```python
from build123d import *

# Parameters (mm, degrees)
SKETCH_1_W          = 0.3
SKETCH_1_H          = 1.5
SKETCH_1_R          = 2.5
SKETCH_1_R_2        = 1.5
EXTRUDE_1_DEPTH     = 15.2
SKETCH_1_4_W        = 0.3
SKETCH_1_4_H        = 1.5
EXTRUDE_2_DEPTH     = 2
CUT_EXTRUDE_2_DEPTH = 19.763794925
FILLET_1_R          = 0.4
SKETCH_1_5_R        = 2.5
SKETCH_1_5_R_2      = 1.5
EXTRUDE_3_DEPTH     = 1.2
CUT_EXTRUDE_START   = -1.2
SKETCH_1_7_R        = 1.5
CUT_EXTRUDE_1_DEPTH = 0.6
FILLET_2_R          = 0.4
SKETCH_3_R          = 2
EXTRUDE_4_DEPTH     = 0.5
SKETCH_3_3_R        = 0.5
EXTRUDE_5_DEPTH     = 6.5


with BuildPart() as part:
    # 草图1 → 凸台-拉伸1 (new body)
    # profile 1 of 5: a face of its own
    with BuildSketch(Plane.XY):
        with BuildLine():
            ThreePointArc((-6, 0), (-5.286764074, -2.837274331), (-3.31662479, -5))
            Line((-3.31662479, -5), (3.31662479, -5))
            ThreePointArc((3.31662479, -5), (5.286764074, -2.837274331), (6, 0))
            ThreePointArc((6, 0), (5.286764074, 2.837274331), (3.31662479, 5))
            Line((3.31662479, 5), (-3.31662479, 5))
            ThreePointArc((-3.31662479, 5), (-5.286764074, 2.837274331), (-6, 0))
        make_face()
        with Locations((-3.65, 0)):
            Rectangle(SKETCH_1_W, SKETCH_1_H, mode=Mode.SUBTRACT)
        Circle(SKETCH_1_R, mode=Mode.SUBTRACT)
        with Locations((3.65, 0)):
            Rectangle(SKETCH_1_W, SKETCH_1_H, mode=Mode.SUBTRACT)
    # profile 2 of 5: a face of its own
    with BuildSketch(Plane.XY):
        Circle(SKETCH_1_R)
        Circle(SKETCH_1_R_2, mode=Mode.SUBTRACT)
    # profile 3 of 5: a face of its own
    with BuildSketch(Plane.XY):
        Circle(SKETCH_1_R_2)
    # profile 4 of 5: a face of its own
    with BuildSketch(Plane.XY):
        with Locations((3.65, 0)):
            Rectangle(SKETCH_1_W, SKETCH_1_H)
    # profile 5 of 5: a face of its own
    with BuildSketch(Plane.XY):
        with Locations((-3.65, 0)):
            Rectangle(SKETCH_1_W, SKETCH_1_H)
    extrude(amount=EXTRUDE_1_DEPTH)

    # 草图1<4> → 凸台-拉伸2 (add)
    with BuildSketch(Plane.XY):
        with Locations((3.65, 0)):
            Rectangle(SKETCH_1_4_W, SKETCH_1_4_H)
        with Locations((-3.65, 0)):
            Rectangle(SKETCH_1_4_W, SKETCH_1_4_H)
    extrude(amount=-EXTRUDE_2_DEPTH)

    # 草图2 → 切除-拉伸2 (cut, through all)
    with BuildSketch(Plane(origin=(3.8, 0, 0), x_dir=(0, 0, -1), z_dir=(1, 0, 0))):
        with BuildLine():
            Line((0.95, 0.45), (1.05, 0.45))
            ThreePointArc((1.05, 0.45), (1.5, 0), (1.05, -0.45))
            Line((1.05, -0.45), (0.95, -0.45))
            ThreePointArc((0.95, -0.45), (0.5, 0), (0.95, 0.45))
        make_face()
    extrude(amount=-CUT_EXTRUDE_2_DEPTH, mode=Mode.SUBTRACT)

    # 圆角1
    fillet_1_edges = [part.edges().sort_by_distance(p)[0] for p in [
        (3.65, -0.75, -2),
        (3.65, 0.75, -2),
        (-3.65, -0.75, -2),
        (-3.65, 0.75, -2),
    ]]
    fillet(fillet_1_edges, radius=FILLET_1_R)

    # 草图1<5> → 凸台-拉伸3 (add)
    # profile 1 of 2: a face of its own
    with BuildSketch(Plane.XY):
        Circle(SKETCH_1_5_R)
        Circle(SKETCH_1_5_R_2, mode=Mode.SUBTRACT)
    # profile 2 of 2: a face of its own
    with BuildSketch(Plane.XY):
        Circle(SKETCH_1_5_R_2)
    extrude(amount=-EXTRUDE_3_DEPTH)

    # 草图1<7> → 切除-拉伸1 (cut)
    with BuildSketch(Plane.XY.offset(CUT_EXTRUDE_START)):
        Circle(SKETCH_1_7_R)
    extrude(amount=CUT_EXTRUDE_1_DEPTH, mode=Mode.SUBTRACT)

    # 圆角2
    fillet_2_edges = [part.edges().sort_by_distance(p)[0] for p in [
        (-2.5, 0, -1.2),
    ]]
    fillet(fillet_2_edges, radius=FILLET_2_R)

    # 草图3 → 凸台-拉伸4 (add)
    with BuildSketch(Plane.XY.offset(15.2)):
        Circle(SKETCH_3_R)
    extrude(amount=EXTRUDE_4_DEPTH)

    # 草图3<3> → 凸台-拉伸5 (add)
    with BuildSketch(Plane.XY.offset(15.2)):
        Circle(SKETCH_3_3_R)
    extrude(amount=EXTRUDE_5_DEPTH)


solid = part.part
```
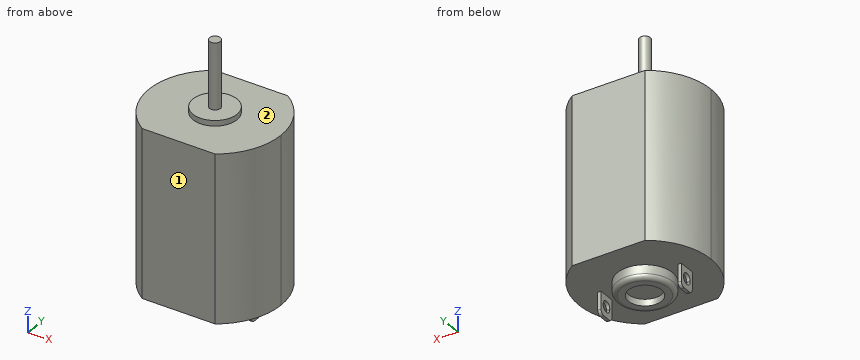
Geometry check sheet. Reference: the model listing, model coordinates, mm. Face numbers are marked on the shaded views. A direction names the side the tool comes from. Give positions to 0.01 mm unless a question says otherwise; leave off trailing zeros. Loops run counter-clockwise (first coordinate to the right, second up) from the corner with the lowest first, then second, coordinate; pieces in that order, holes last. Notation, with made-up numbers: M 53,51 L 58,51 A24 ccw 58,73 Z; hole C 68,66 d3. An arc over 180 degrees is marked long. Write item = value, one per line.
(1) Tool access check on the marked faces 1 and 2. Record the directions out of +Z, -Z, +X, -X, +Y, -Y that give a thin tool (end or side, any length) a straight path to the whole face; none if there is none.
Answer below:
face_1 = +Z, -Z, +X, -X, -Y
face_2 = +Z
(2) Sectioned sample at D-D, the plane x = 5. Record the cut outline in (y, z), plus the area to 3 significant figures.
Answer below:
outline = M -3.32,0 L 3.32,0 L 3.32,15.2 L -3.32,15.2 Z
area = 101 mm2
(3) Gauge pin test, flat ends, axial feed: pin 1 Ø2 at (x, y) = (3, -2) entering from +Z; pin 2 Ø2 at (x, y) = (1, 0.5) entering from -Z; pin 3 Ø1.2 at (y, z) = (-0.5, -0.5) entering from -X; pin 4 Ø6 at (x, y) = (1.5, 1) entering from +Z. Record the tip position at first contact, or that the pin passes through.
Answer below:
pin_1 = 15.2
pin_2 = -1.2
pin_3 = -6
pin_4 = 21.7
(4) Sectioned sample at B-B, the plane z = 14.5. Record the cut outline in (x, y).
Answer below:
outline = M -3.32,-5 L 3.32,-5 A6 ccw 3.32,5 L -3.32,5 A6 ccw Z
(5) Sectioned sample at A-A, the plane x = 0. Record the cut outline in (y, z).
Answer below:
outline = M -5,0 L -2.5,0 L -2.5,-0.8 A0.4 ccw -2.1,-1.2 L -1.5,-1.2 L -1.5,-0.6 L 1.5,-0.6 L 1.5,-1.2 L 2.1,-1.2 A0.4 ccw 2.5,-0.8 L 2.5,0 L 5,0 L 5,15.2 L 2,15.2 L 2,15.7 L 0.5,15.7 L 0.5,21.7 L -0.5,21.7 L -0.5,15.7 L -2,15.7 L -2,15.2 L -5,15.2 Z
(6) Material ranges on line 1 (Z direction, x = 3.25, y = 4.25); line 2 (Z direction, x = -1.5, y = 0.5); line 3 (Y direction, x = 0, z = -1.1), recorded low to high. Write a range as [from, to].
Answer below:
line_1 = [0, 15.2]
line_2 = [-1.2, 15.7]
line_3 = [-2.36, -1.5], [1.5, 2.36]
(7) Sectioned sample at C-C, the plane y = 4.75. Record the cut outline in (x, z).
Answer below:
outline = M -3.67,0 L 3.67,0 L 3.67,15.2 L -3.67,15.2 Z
